The model under review builds one solid part; all positions refer to its coordinate system, in mm. A direction names the side the tool comes from. Round coordinates to 2 decimals unless told otherwise and drop trailing zeros. Loops run counter-clockwise (first coordinate to the right, second up) from the corner with the lowest first, then second, coordinate; pieces in that order, holes last. Notation, with made-up numbers: M -24.5,0.5 L 12.5,0.5 A29 cw 12.5,35.5 Z; hole C -24,40 d2. An arc over 180 degrees is marked long. Return JSON: item names as keys, results as strings. Group by question number.
Q1. Draft analysis for pull direction Z (two halves, no side actions). For faces 5 (the face through (-12, -10, -5)), 6 (the face through (-34, 0, -1)), 7 (the face through (-1, -80, 75)), 8 (the face through (-1, -15, -75)), state which applies: pulls with the +Z half, pulls with the -Z half, needs draft (parallel to the pull), parting line crosses it, or undercut.
Q2. Consider section C-C (y = -21.5). Count the separate pieces of the cut face and the enclosed holes in it, and give its area (3 significant figures).
Q3. Clearance check with flat-ended pins moving along their axes: pin 1 Ø12 at (x, y) = (-50, -46.5) entering from -Z; pin 2 Ø10 at (x, y) = (30, -43.5) entering from -Z; pin 3 Ø11 at (y, z) = (-46, -15) entering from -X; pin 4 Ø18.5 at (y, z) = (-60.5, -12) entering from +X. State where each tip first meets the part, or that it passes through.
Q4. Consider section A-A (x = 49). State the section outline as (y, z) points.
Q5. For faces 1 (the face through (63.763, -15.21, 55.989)), 2 (the face through (-65, -82, 2)), 3 (the face through (-1, -30, -51)), 4 (the face through (40, -51, -1)), list the 3-axis set-ups (+Z, -Z, +X, -X, +Y, -Y) from which the entire face can be reached by the end or side of a thin tool; tool diameter is ignored.
Q6. To check wall thickness, follow line 1 along Z through (x, y) = (-60, -21); line 2 along X through (y, z) = (-16.5, 2); line 3 along Y through (x, z) = (68, 4). State the ranges of each line that lie inside material, in increasing order.
Q7. Consider section B-B (y = -43). State the section outline as (x, z) points.
from build123d import *

# Parameters (mm, degrees)
IZIM2_W                     = 150
IZIM2_H                     = 150
Y_KSEKLIK_EKSTR_ZYON1_DEPTH = 30
IZIM3_W                     = 80
IZIM3_H                     = 80
Y_KSEKLIK_EKSTR_ZYON2_DEPTH = 40
IZIM5_W                     = 150
IZIM5_H                     = 150
Y_KSEKLIK_EKSTR_ZYON3_DEPTH = 20
DELIK4_D                    = 27
DELIK4_CBORE_D              = 60
DELIK4_CBORE_DEPTH          = 10
M16_START                   = -30
M16_DI_LI_DELIK1_OUTLINE_R  = 7
M16_DI_LI_DELIK1_DEPTH      = 30
F_10_0_10_AP_DELIK1_D       = 10
F_10_0_10_AP_DELIK1_DEPTH   = 14.995696905
F_10_0_10_AP_DELIK1_TIP     = 3.004303095
RADYUS1_R                   = 3
RADYUS2_R                   = 2


# Read off the part's stored shape, not the designer's step: M16 Dişli Delik1
with BuildPart() as part:
    # Çizim2 → Yükseklik-Ekstrüzyon1 (new body)
    with BuildSketch(Plane(origin=(0, 0, 0), x_dir=(1, 0, 0), z_dir=(0, 1, 0))):
        Rectangle(IZIM2_W, IZIM2_H)
    extrude(amount=-Y_KSEKLIK_EKSTR_ZYON1_DEPTH)

    # Çizim3 → Yükseklik-Ekstrüzyon2 (add)
    with BuildSketch(Plane.XZ.offset(30)):
        Rectangle(IZIM3_W, IZIM3_H)
    extrude(amount=Y_KSEKLIK_EKSTR_ZYON2_DEPTH)

    # Çizim5 → Yükseklik-Ekstrüzyon3 (add)
    with BuildSketch(Plane.XZ.offset(70)):
        Rectangle(IZIM5_W, IZIM5_H)
    extrude(amount=Y_KSEKLIK_EKSTR_ZYON3_DEPTH)

    # Delik4 (through all)
    with Locations(Plane(origin=(0, 0, 1.891621306), x_dir=(0, 0, 1), z_dir=(0, 1, 0))):
        with Locations((0, 0)):
            CounterBoreHole(DELIK4_D / 2, DELIK4_CBORE_D / 2, DELIK4_CBORE_DEPTH)

    # M16 Dişli Delik1 outline → M16 Dişli Delik1 (cut)
    with BuildSketch(Plane(origin=(0, 0, 0), x_dir=(1, 0, 0), z_dir=(0, 1, 0)).offset(M16_START)):
        with Locations((0, -61.891621306)):
            Circle(M16_DI_LI_DELIK1_OUTLINE_R)
        with Locations((60, -1.891621306)):
            Circle(M16_DI_LI_DELIK1_OUTLINE_R)
        with Locations((-60, -1.891621306)):
            Circle(M16_DI_LI_DELIK1_OUTLINE_R)
        with Locations((0, 58.108378694)):
            Circle(M16_DI_LI_DELIK1_OUTLINE_R)
        with Locations((60, 58.108378694)):
            Circle(M16_DI_LI_DELIK1_OUTLINE_R)
        with Locations((-60, -61.891621306)):
            Circle(M16_DI_LI_DELIK1_OUTLINE_R)
        with Locations((-60, 58.108378694)):
            Circle(M16_DI_LI_DELIK1_OUTLINE_R)
        with Locations((60, -61.891621306)):
            Circle(M16_DI_LI_DELIK1_OUTLINE_R)
    extrude(amount=M16_DI_LI_DELIK1_DEPTH, mode=Mode.SUBTRACT)

    # Ø10.0 (10) Çap Delik1
    with Locations(Plane(origin=(0, -90, 0), x_dir=(-1, 0, 0), z_dir=(0, -1, 0))):
        with Locations((0, -1.891621306), (0, 58.108378694), (-60, -1.891621306), (60, -1.891621306), (0, -61.891621306)):
            Hole(F_10_0_10_AP_DELIK1_D / 2, depth=F_10_0_10_AP_DELIK1_DEPTH)
            with Locations((0, 0, -(F_10_0_10_AP_DELIK1_DEPTH + F_10_0_10_AP_DELIK1_TIP / 2))):  # 118° drill point
                Cone(0, F_10_0_10_AP_DELIK1_D / 2, F_10_0_10_AP_DELIK1_TIP, mode=Mode.SUBTRACT)

    # Radyus1
    radyus1_edges = [part.edges().sort_by_distance(p)[0] for p in [
        (40, -30, 0),
        (0, -30, 40),
        (-40, -30, 0),
        (0, -30, -40),
    ]]
    fillet(radyus1_edges, radius=RADYUS1_R)

    # Radyus2
    radyus2_edges = [part.edges().sort_by_distance(p)[0] for p in [
        (0, -10, -28.108378694),
    ]]
    fillet(radyus2_edges, radius=RADYUS2_R)


solid = part.part
Values:
{
 "1": {"face 5": "undercut", "face 6": "needs draft", "face 7": "pulls with the +Z half", "face 8": "pulls with the -Z half"},
 "2": {"separate pieces": "1", "enclosed holes": "9", "area": "20,700 mm2"},
 "3": {"pin 1": "passes through", "pin 2": "stops at z = -40", "pin 3": "stops at x = -40", "pin 4": "stops at x = 40"},
 "4": {"outline": "M -90,-75 L -70,-75 L -70,75 L -90,75 Z; M -30,-75 L 0,-75 L 0,75 L -30,75 Z"},
 "5": {"face 1": "+Y", "face 2": "-Y", "face 3": "none", "face 4": "+Z, -Z, +X"},
 "6": {"line 1": "z = -75 to -65.11, -51.11 to -5.11, 8.89 to 54.89, 68.89 to 75", "line 2": "x = -75 to -67, -53 to -13.5, 13.5 to 53, 67 to 75", "line 3": "y = -90 to -70, -30 to 0"},
 "7": {"outline": "M -40,-40 L 40,-40 L 40,40 L -40,40 Z; hole C 0,1.89 d27"}
}
